Check sheet for the drawn part. Datum: minimum x, y, z corner. Units: mm. Give positions to 0.01 mm unless a question says otherwise; leave off trailing zeros. Loops run counter-clockwise (first coordinate to the right, second up) from the corner with the lowest first, then second, coordinate; pieces in that order, holes last. Notation, with made-up numbers: (-21, -19) -> (37, -19) arc R20 cw to (37, -11) -> close; hole circle Ø11 at (51.25, -2). An arc over 180 degrees is marked (long way). One line per question, with ' | ' between items.
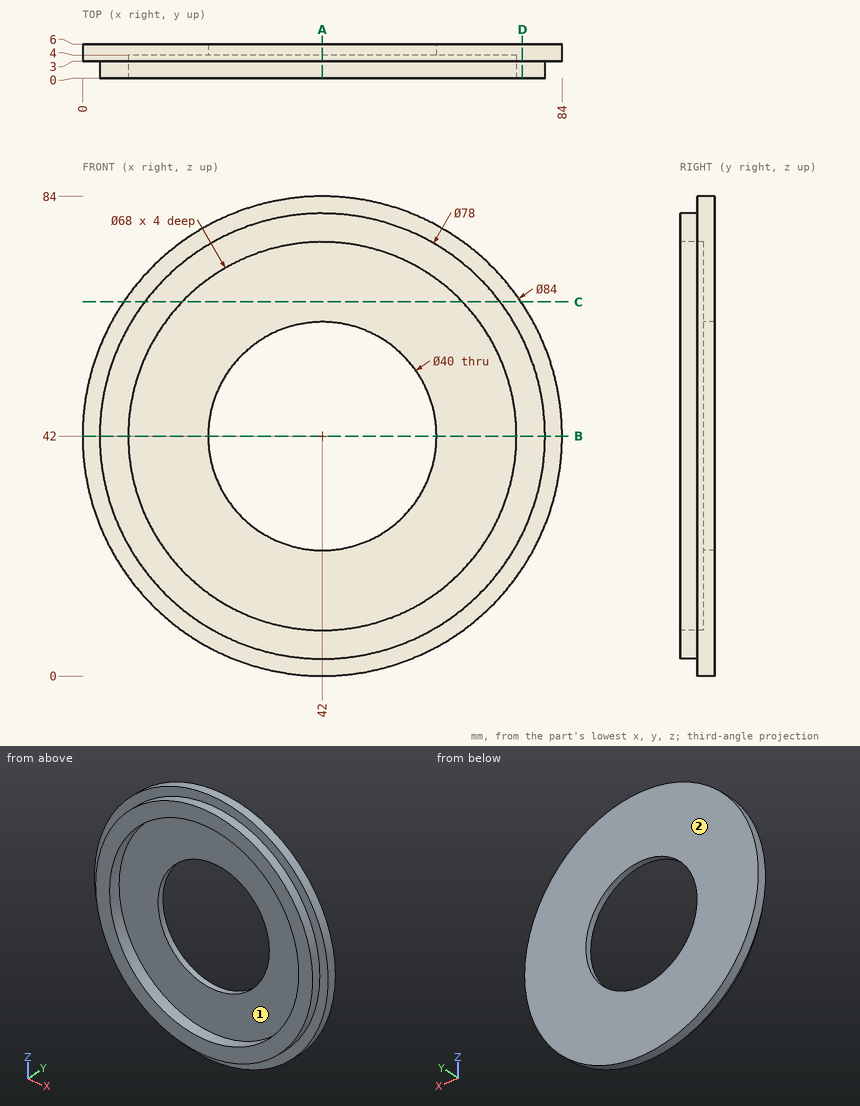
Item 1: Sectioned sample at A-A (x = 42). Record the cut outline in (y, z), plus the area to 3 significant figures.
Result:
outline: (0, 3) -> (3, 3) -> (3, 0) -> (6, 0) -> (6, 22) -> (4, 22) -> (4, 8) -> (0, 8) -> close; (0, 76) -> (4, 76) -> (4, 62) -> (6, 62) -> (6, 84) -> (3, 84) -> (3, 81) -> (0, 81) -> close | area: 134 mm2
Item 2: Scan lines: probe 1 along Z at (x, y) = (42, 5.5); probe 2 along Z at (x, y) = (42, 3.1); probe 3 along Y at (x, z) = (36.5, 62.5). Record each from-to range of solid material in increasing order.
Result:
probe 1: 0 to 22, 62 to 84 | probe 2: 0 to 8, 76 to 84 | probe 3: 4 to 6
Item 3: Sectioned sample at C-C (z = 65.5). Record the cut outline in (x, y).
Result:
outline: (7.19, 3) -> (10.88, 3) -> (10.88, 0) -> (17.43, 0) -> (17.43, 4) -> (66.57, 4) -> (66.57, 0) -> (73.12, 0) -> (73.12, 3) -> (76.81, 3) -> (76.81, 6) -> (7.19, 6) -> close
Item 4: Sectioned sample at B-B (z = 42). Record the cut outline in (x, y).
Result:
outline: (0, 3) -> (3, 3) -> (3, 0) -> (8, 0) -> (8, 4) -> (22, 4) -> (22, 6) -> (0, 6) -> close; (62, 4) -> (76, 4) -> (76, 0) -> (81, 0) -> (81, 3) -> (84, 3) -> (84, 6) -> (62, 6) -> close
Item 5: Release check for a two-part mould opening along Z. For the marked faces 1 and 2 record: pulls with the +Z half, pulls with the -Z half, needs draft (parallel to the pull), parting line crosses it, or undercut.
Result:
face 1: undercut | face 2: needs draft
Item 6: Sectioned sample at D-D (x = 77). Record the cut outline in (y, z).
Result:
outline: (0, 24.8) -> (3, 24.8) -> (3, 18.78) -> (6, 18.78) -> (6, 65.22) -> (3, 65.22) -> (3, 59.2) -> (0, 59.2) -> close
Item 7: Depth check by flat-ended pin: pin 1 Ø2 at (x, y) = (49.5, 5) entering from +Z; pin 2 Ø3 at (y, z) = (1, 35) entering from -X; pin 3 Ø8 at (x, z) = (37, 71) entering from -Y. Enter the tip coordinate at first touch or a pass-through.
Result:
pin 1: z = 83.49 | pin 2: x = 3.39 | pin 3: y = 4
